```python
from build123d import *

# Parameters (mm, degrees)
SKETCH1_W                         = 116
SKETCH1_H                         = 100
BOSS_EXTRUDE1_DEPTH               = 3
TAP_DRILL_FOR_M3_TAP1_D           = 2.5
TAP_DRILL_FOR_M3_TAP1_CSINK_D     = 2.55
TAP_DRILL_FOR_M3_TAP1_CSINK_ANGLE = 90


with BuildPart() as part:
    # Sketch1 → Boss-Extrude1 (new body)
    with BuildSketch(Plane(origin=(0, 0, 0), x_dir=(1, 0, 0), z_dir=(0, 1, 0))):
        Rectangle(SKETCH1_W, SKETCH1_H)
    extrude(amount=BOSS_EXTRUDE1_DEPTH)

    # Tap Drill for M3 Tap1 (through all)
    with Locations(Plane(origin=(0, 3, 0), x_dir=(1, 0, 0), z_dir=(0, 1, 0))):
        with Locations((0, 29.5), (-54, -38.5), (54, -38.5)):
            CounterSinkHole(TAP_DRILL_FOR_M3_TAP1_D / 2, TAP_DRILL_FOR_M3_TAP1_CSINK_D / 2, counter_sink_angle=TAP_DRILL_FOR_M3_TAP1_CSINK_ANGLE)


solid = part.part
```
Read the model definition and answer for the solid it produces. Units are mm, in the model's axes. Coordinates: 2 decimals unless noted, no trailing zeros. Order: outer loops, then holes, each group sorted by start corner. A loop starts at its lowest first (then second) coordinate and runs counter-clockwise, first axis right, second up. Notation, with made-up numbers: (33.5, 79) - (75.5, 79) arc R26 ccw to (75.5, 107) - close; hole circle Ø2 at (-29, -24.5). An arc over 180 degrees is marked (long way). Answer as a JSON object with one key per item and string values. Group by question number.
Item 1: Section B-B (x = 0) is taken. Give the vertices of the cut face in (y, z) (3 decimals), plus the area to 4 significant figures.
Item 2: The mould has two halves that part along X. Classify faces 1 (the face through (-55.155, 1.467, 38.979)), 2 (the face through (-58, 1, 1)), 3 (the face through (-1, 1, -50)): +X half, -X half, draft (parallel to the pull), parting line (faces both ways), or undercut.
Item 3: Section C-C (z = 38.5) is taken. Give the vertices of the cut face in (x, y) (3 decimals).
Item 4: Section A-A (z = -29.5) is taken. Give the vertices of the cut face in (x, y) (3 decimals), plus the area to 4 significant figures.
Item 5: Consider probe 1 along X at (y, z) = (1.9, 38.5); probe 2 along Z at (x, y) = (54, 0.8); probe 3 along X at (y, z) = (0.6, 39.5). Determine where each line is inside the solid, lowest interval first. Write a range as from..to.
Results are:
{
 "1": {"outline": "(0, -50) - (3, -50) - (3, -30.775) - (2.975, -30.75) - (0, -30.75) - close; (0, -28.25) - (2.975, -28.25) - (3, -28.225) - (3, 50) - (0, 50) - close", "area": "292.5 mm^2"},
 "2": {"face 1": "undercut", "face 2": "-X half", "face 3": "draft"},
 "3": {"outline": "(-58, 0) - (-55.25, 0) - (-55.25, 2.975) - (-55.275, 3) - (-58, 3) - close; (-52.75, 0) - (52.75, 0) - (52.75, 2.975) - (52.725, 3) - (-52.725, 3) - (-52.75, 2.975) - close; (55.25, 0) - (58, 0) - (58, 3) - (55.275, 3) - (55.25, 2.975) - close"},
 "4": {"outline": "(-58, 0) - (-1.25, 0) - (-1.25, 2.975) - (-1.275, 3) - (-58, 3) - close; (1.25, 0) - (58, 0) - (58, 3) - (1.275, 3) - (1.25, 2.975) - close", "area": "340.5 mm^2"},
 "5": {"probe 1": "x = -58..-55.25, -52.75..52.75, 55.25..58", "probe 2": "z = -50..37.25, 39.75..50", "probe 3": "x = -58..-54.75, -53.25..53.25, 54.75..58"}
}
